CAD build for the part. Positions are in the model's coordinates, mm. Give positions to 0.01 mm unless a question says otherwise; leave off trailing zeros. Order: outer loops, then holes, each group sorted by start corner. A loop starts at its lowest first (then second) coordinate and runs counter-clockwise, first axis right, second up. Notation, with made-up numbers: M 75,-35.5 L 126,-35.5 A23 cw 126,-23.5 Z; hole C 76,-24 d7. An arc over 180 degrees is marked long. Put each result on its own line as item: value. Start each with the question number.
1) Two-plate mould, pull along X, no slides. Class faces 1 (the face through (-14.985, 0.66, 1.696)), 2 (the face through (0, 0, 2)), 3 (the face through (0, 0, 0)): released by +X, released by -X, zero draft, split by the parting line, or undercut.
2) Pin check, flat tips, straight feed: pin 1 (1.5 mm diameter, centred on x = -4.5, z = 5.5, fed in from +Y); pin 2 (3 mm diameter, centred on x = -9.5, z = 5, fed in from -Y); pin 3 (1 mm diameter, centred on x = -10.5, z = 3, fed in from -Y). Stop position of each tip, or through.
3) Cut at C-C (z = 4). Write the cut outline in (x, y).
4) Cut at D-D (z = 1). Write the cut outline in (x, y), and give its area (3 significant figures).
5) Drill centre lines: line 1 (Y direction, x = -8.5, z = 5.75); line 2 (X direction, y = -4.5, z = 3.75); line 3 (Z direction, x = -0.25, y = -3). Where is each one in solid material? Low to high. Write a range as [from, to].
```python
from build123d import *

# Parameters (mm, degrees)
F0_R     = 15
F0_R_2   = 13
F0_R_3   = 12.6
F0_R_4   = 11
F1_DEPTH = 2
F2_DEPTH = 7
F3_R     = 4.99999
F4_SIZE  = 1.4
F5_R     = 1.4


# Not quite as in the source:
# - a fillet or chamfer is up to 0.001 mm smaller than in the source, because OpenCascade refuses the exact size


with BuildPart() as f1:
    # F0 (on Top) → F1 (new body)
    with BuildSketch(Plane.XY):
        Circle(F0_R)
        Circle(F0_R_2, mode=Mode.SUBTRACT)
        Circle(F0_R_2)
        Circle(F0_R_3, mode=Mode.SUBTRACT)
        Circle(F0_R_3)
        Circle(F0_R_4, mode=Mode.SUBTRACT)
        Circle(F0_R_4)
    extrude(amount=F1_DEPTH)

    # F0 (on Top) → F2 (join)
    with BuildSketch(Plane.XY):
        Circle(F0_R_3)
        Circle(F0_R_4, mode=Mode.SUBTRACT)
    extrude(amount=F2_DEPTH)

    # F3 (radius 5 in the source; OpenCascade refuses exactly that, so slightly less here)
    f3_edges = [f1.edges().sort_by_distance(p)[0] for p in [
        (-11, 0, 2),
    ]]
    fillet(f3_edges, radius=F3_R)

    # F4
    f4_edges = [f1.edges().sort_by_distance(p)[0] for p in [
        (-12.6, 0, 7),
    ]]
    chamfer(f4_edges, length=F4_SIZE)

    # F5
    f5_edges = [f1.edges().sort_by_distance(p)[0] for p in [
        (-15, 0, 0),
    ]]
    fillet(f5_edges, radius=F5_R)


solid = f1.part
```
Solution:
1. face 1: split by the parting line
1. face 2: undercut
1. face 3: zero draft
2. pin 1: y = 12.03
2. pin 2: y = -9.73
2. pin 3: y = -7.67
3. outline: C 0,0 d25.2; hole C 0,0 d20
4. outline: C 0,0 d29.88
4. area: 701 mm²
5. line 1: [-9.1, -6.73], [6.73, 9.1]
5. line 2: [-11.77, -8.71], [8.71, 11.77]
5. line 3: [0, 2]
